from build123d import *

# Parameters (mm, degrees)
FASE1_SIZE                      = 0.25
AUFSATZ_LINEAR_AUSTRAGEN1_DEPTH = 5


with BuildPart() as part:
    # Skizze1 → Rotation1 (revolve)
    with BuildSketch(Plane.XY):
        Polygon((-8, 3), (-11, 3), (-11, 0), (0, 0), (0, 2.5), (-4, 2.5), (-4, 3.5), (-4.5, 3.5), (-4.5, 5), (-5, 5), (-5.5, 4.5), (-6.5, 4.5), (-7, 5), (-7.5, 5), (-7.5, 3.5), (-8, 3.5), align=None)
    revolve(axis=Axis((-5.518776228, 0, 0), (-1, 0, 0)))

    # Fase1
    fase1_edges = [part.edges().sort_by_distance(p)[0] for p in [
        (-4.5, -5, 0),
        (-7.5, -5, 0),
    ]]
    chamfer(fase1_edges, length=FASE1_SIZE)

    # Spiegeln1: part across plane


with BuildPart() as part_1:
    add(part.part)
    add(part.part.mirror(Plane(origin=(0, 0, 0), x_dir=(0, 0, 1), z_dir=(1, 0, 0))))

    # Skizze2 → Aufsatz-Linear austragen1 (add)
    with BuildSketch(Plane.ZY.offset(11)):
        with BuildLine():
            Line((-0.5, -1.936491673), (-0.5, -2.907318352))
            ThreePointArc((-0.5, -2.907318352), (-2.95, 0), (-0.5, 2.907318352))
            Line((-0.5, 2.907318352), (-0.5, 1.936491673))
            ThreePointArc((-0.5, 1.936491673), (-2, 0), (-0.5, -1.936491673))
        make_face()
        with BuildLine():
            Line((0.5, -1.936491673), (0.5, -2.907318352))
            ThreePointArc((0.5, -2.907318352), (2.95, 0), (0.5, 2.907318352))
            Line((0.5, 2.907318352), (0.5, 1.936491673))
            ThreePointArc((0.5, 1.936491673), (2, 0), (0.5, -1.936491673))
        make_face()
    extrude(amount=AUFSATZ_LINEAR_AUSTRAGEN1_DEPTH)


solid = part_1.part
The model under review builds one solid part; all positions refer to its coordinate system, in mm. A direction names the side the tool comes from. Round coordinates to 2 decimals unless told otherwise and drop trailing zeros. Loops run counter-clockwise (first coordinate to the right, second up) from the corner with the lowest first, then second, coordinate; pieces in that order, holes last. Notation, with made-up numbers: (-13, -28) -> (45, -28) arc R18 ccw to (45, 7) -> close; hole circle Ø6 at (88.5, 37.25). An arc over 180 degrees is marked (long way). Write item = value, one per line. Start each with the question number.
Item 1: To check wall thickness, follow L1, parallel to X at y = -2, z = -2; L2, parallel to X at y = 0.5, z = -3.75; L3, parallel to Y at x = 1.75, z = 0. State the ranges of each line that lie inside material, in increasing order.
Item 2: Mouldability with a two-part tool opening along Y and no side actions: class faces 1 (the cylindrical face through (-13, 0, -2)), 2 (the cylindrical face through (10, -3, 0)), 3 (the flat face through (-4.5, 4, 0)) as released by +Y, released by -Y, zero draft, split by the parting line, or undercut.
Item 3: Take a section at C-C on x = 3.5. Give the boundary of the cut face in (y, z).
Item 4: Take a section at B-B on x = -8.25. Give the boundary of the cut face in (y, z).
Item 5: Take a section at A-A on x = -12.5. Give the boundary of the cut face in (y, z), plus the area to 3 significant figures.
Item 6: Insertion check: pin 1 (2 mm diameter, centred on y = -0.5, z = -0.5, fed in from -X); pin 2 (1.5 mm diameter, centred on y = 3.5, z = -4, fed in from -X); pin 3 (1.1 mm diameter, centred on x = -13.5, y = 2.5, fed in from -Z). Each pin has a flat end and moves straight along its axis. Give the tip position at first contact, or say it passes through.
Item 7: For faces 4 (the cylindrical face through (-10, -3, 0)), 5 (the flat face through (8, 3, -1)), 6 (the cylindrical face through (-6.01, -0.59, -4.46)), 7 (the flat face through (-13.5, -2.4, 0.5)), list the 3-axis set-ups (+Z, -Z, +X, -X, +Y, -Y) from which the entire face can be reached by the end or side of a thin tool; tool diameter is ignored.
Result:
q1.L1 = -16 to -4, 4 to 11
q1.L2 = -7.5 to -4.5, 4.5 to 7.5
q1.L3 = -2.5 to 2.5
q2.face_1 = undercut
q2.face_2 = split by the parting line
q2.face_3 = zero draft
q3.outline = circle Ø5 at (0, 0)
q4.outline = circle Ø6 at (0, 0)
q5.outline = (-2.91, -0.5) arc R2.95 ccw to (2.91, -0.5) -> (1.94, -0.5) arc R2 cw to (-1.94, -0.5) -> close; (-2.91, 0.5) -> (-1.94, 0.5) arc R2 cw to (1.94, 0.5) -> (2.91, 0.5) arc R2.95 ccw to start
q5.area = 12.9 mm²
q6.pin_1 = -11
q6.pin_2 = -7.5
q6.pin_3 = -2.21
q7.face_4 = -X
q7.face_5 = +X
q7.face_6 = none
q7.face_7 = -X, +Y, -Y
